Read the model definition and answer for the solid it produces. Units are mm, in the model's axes. A direction names the side the tool comes from. Coordinates: 2 decimals unless noted, no trailing zeros. Order: outer loops, then holes, each group sorted by start corner. A loop starts at its lowest first (then second) coordinate and runs counter-clockwise, first axis right, second up.
```python
from build123d import *

# Parameters (mm, degrees)
SKETCH1_W               = 30
SKETCH1_H               = 110
BOSS_EXTRUDE1_DEPTH     = 5
SKETCH3_R               = 5
BOSS_EXTRUDE3_DEPTH     = 110
CUT_EXTRUDE3_DEPTH      = 123.576506721
CUT_EXTRUDE3_DEPTH_BACK = 123.576506721
SKETCH5_W               = 40
SKETCH5_H               = 90


with BuildPart() as part:
    # Sketch1 → Boss-Extrude1 (new body)
    with BuildSketch(Plane.XY):
        with Locations((15, 55)):
            Rectangle(SKETCH1_W, SKETCH1_H)
    extrude(amount=BOSS_EXTRUDE1_DEPTH)

    # Sketch3 → Boss-Extrude3 (add, through all)
    with BuildSketch(Plane(origin=(0, 110, 0), x_dir=(1, 0, 0), z_dir=(0, 1, 0))):
        with BuildLine():
            Line((0, -5), (0, -35.031831765))
            ThreePointArc((0, -35.031831765), (2.65246331, -41.815171989), (9.202740917, -45))
            ThreePointArc((9.202740917, -45), (16.121762832, -41.525252064), (20.338661017, -35.031831765))
            Line((20.338661017, -35.031831765), (30, -5))
            Line((30, -5), (0, -5))
        make_face()
        with Locations(Location((10, -35.031831765, 0), (0, 0, 270))):
            Circle(SKETCH3_R, mode=Mode.SUBTRACT)
    extrude(amount=-BOSS_EXTRUDE3_DEPTH)

    # Sketch5 → Cut-Extrude3 (cut, two sides: drawn at the far end of the back side and taken through both)
    with BuildSketch(Plane(origin=(0, 0, 0), x_dir=(0, 0, -1), z_dir=(1, 0, 0)).offset(-CUT_EXTRUDE3_DEPTH_BACK)):
        with Locations((-25, 55)):
            Rectangle(SKETCH5_W, SKETCH5_H)
    extrude(amount=CUT_EXTRUDE3_DEPTH + CUT_EXTRUDE3_DEPTH_BACK, mode=Mode.SUBTRACT)


solid = part.part
```
1) Determine the mould class of faces 1 (the flat face through (15, 54, 5)), 2 (the cylindrical face through (10.22, 105.07, 30.037)), 3 (the flat face through (11, 0, 17)) for opening direction Y: pulls with the +Y half, pulls with the -Y half, needs draft (parallel to the pull), parting line crosses it, or undercut.
A:
face 1: undercut
face 2: needs draft
face 3: pulls with the -Y half
2) A cutting plane is placed at D-D, the plane x = 17. Determine the outline of the cut face in (y, z), and give its area (3 significant figures).
A:
outline: (0, 0) - (110, 0) - (110, 40.67) - (100, 40.67) - (100, 5) - (10, 5) - (10, 40.67) - (0, 40.67) - close
area: 1,260 mm2
3) A cutting plane is placed at B-B, the plane z = 29. Determine the outline of the cut face in (x, y), and give its area (3 significant figures).
A:
outline: (0, 0) - (22.28, 0) - (22.28, 10) - (0, 10) - close; (0, 100) - (22.28, 100) - (22.28, 110) - (0, 110) - close
area: 446 mm2
4) Flat-ended cylindrical pins translate along their axes: pin 1 Ø3 at (x, y) = (3, 99) entering from +Z; pin 2 Ø9 at (x, z) = (10, 35.03) entering from +Y; pin 3 Ø1 at (x, y) = (21, 90.5) entering from +Z. Find the tip coordinate at first contact, or state that the pin passes through.
A:
pin 1: stops at z = 43.12
pin 2: passes through
pin 3: stops at z = 5
5) A cutting plane is placed at A-A, the plane x = 11.5. Determine the outline of the cut face in (y, z), and give its area (3 significant figures).
A:
outline: (0, 0) - (110, 0) - (110, 30.26) - (100, 30.26) - (100, 5) - (10, 5) - (10, 30.26) - (0, 30.26) - close; (0, 39.8) - (10, 39.8) - (10, 44.34) - (0, 44.34) - close; (100, 39.8) - (110, 39.8) - (110, 44.34) - (100, 44.34) - close
area: 1,150 mm2
6) A cutting plane is placed at C-C, the plane z = 36.5. Determine the outline of the cut face in (x, y), and give its area (3 significant figures).
A:
outline: (0.11, 0) - (5.22, 0) - (5.22, 10) - (0.11, 10) - close; (0.11, 100) - (5.22, 100) - (5.22, 110) - (0.11, 110) - close; (14.78, 0) - (19.78, 0) - (19.78, 10) - (14.78, 10) - close; (14.78, 100) - (19.78, 100) - (19.78, 110) - (14.78, 110) - close
area: 202 mm2
7) Which of the six approach directions +Z, -Z, +X, -X, +Y, -Y give full straight-line access (tool end or side, diameter ignored) to faces 4 (the flat face through (25.1, 5.07, 20.23)), 5 (the flat face through (11, 100, 21))?
A:
face 4: +Z, +X, +Y, -Y
face 5: +Z, +X, -X
8) Straight lines are drawn through the part: line 1 (Y direction, x = 2, z = 28.5); line 2 (Z direction, x = 23, y = 25); line 3 (Z direction, x = 11, y = 102.5). For each, find the intervals that lie inside material, in ascending order.
A:
line 1: y = 0 to 10, 100 to 110
line 2: z = 0 to 5
line 3: z = 0 to 30.13, 39.93 to 44.51
